Read the model definition and answer for the solid it produces. Units are mm, in the model's axes. A direction names the side the tool comes from. Round coordinates to 2 decimals unless told otherwise and drop trailing zeros. Write each loop counter-clockwise with the first axis right and the second up, starting at its lowest first coordinate (ties: lowest second). Pieces come first, ordered by that corner, then holes.
from build123d import *

# Parameters (mm, degrees)
BOSS_EXTRUDE1_DEPTH = 6
SKETCH2_W           = 6
SKETCH2_H           = 3


with BuildPart() as part:
    # Sketch1 → Boss-Extrude1 (new body)
    with BuildSketch(Plane(origin=(0, 0, 0), x_dir=(0, 0, -1), z_dir=(1, 0, 0))):
        Polygon((0, 5.773502692), (-5, 2.886751346), (-5, -2.886751346), (0, -5.773502692), (5, -2.886751346), (5, 2.886751346), align=None)
    extrude(amount=-BOSS_EXTRUDE1_DEPTH)

    # Sketch2 → Cut-Revolve4 (revolve, cut)
    with BuildSketch(Plane.XY):
        Polygon((0, 5), (-0.446581987, 5.773502692), (0, 5.773502692), align=None)
        with BuildLine():
            Line((-3.553418013, 5.773502692), (-4, 5))
            Line((-4, 5), (-5, 5))
            ThreePointArc((-5, 5), (-5.707106781, 4.707106781), (-6, 4))
            Line((-6, 4), (-6.773502692, 4))
            Line((-6.773502692, 4), (-6.773502692, 5.773502692))
            Line((-6.773502692, 5.773502692), (-3.553418013, 5.773502692))
        make_face()
        with Locations((-3, 1.5)):
            Rectangle(SKETCH2_W, SKETCH2_H)
    revolve(axis=Axis((-8.121993413, 0, 0), (1, 0, 0)), mode=Mode.SUBTRACT)


solid = part.part
Q1. Determine the mould class of faces 3 (the cylindrical face through (-3, -3, 0)), 4 (the conical face through (-3.894, 2.603, 4.483)), 5 (the flat face through (-1.972, -4.35, -2.465)), 6 (the flat face through (0, 0.1, -3.3)) for opening direction Y: pulls with the +Y half, pulls with the -Y half, needs draft (parallel to the pull), parting line crosses it, or undercut.
Verdict:
face 3: undercut
face 4: pulls with the +Y half
face 5: pulls with the -Y half
face 6: needs draft
Q2. Which of the six approach directions +Z, -Z, +X, -X, +Y, -Y give full straight-line access (tool end or side, diameter ignored) to faces 1 (the cylindrical face through (-4.51, -1.08, -4.88)), 2 (the flat face through (-1.972, -4.31, 2.535))?
Verdict:
face 1: -X
face 2: +Z, +X, -X, -Y
Q3. Straight lines are drawn through the part: probe 1 along Z at (x, y) = (-3.15, 0); probe 2 along Y at (x, z) = (-4.2, 2); probe 3 along Z at (x, y) = (-4.2, 2.25). For each, find the intervals that lie inside material, in ascending order.
Verdict:
probe 1: z = -5 to -3, 3 to 5
probe 2: y = -4.58 to -2.24, 2.24 to 4.58
probe 3: z = -4.47 to -1.98, 1.98 to 4.47
Q4. Section A-A (x = -2.4) is taken. Determine the outline of the cut face in (y, z), then the cut area to 3 significant figures.
Verdict:
outline: (-5.77, 0) - (-2.89, -5) - (2.89, -5) - (5.77, 0) - (2.89, 5) - (-2.89, 5) - close; hole circle Ø6 at (0, 0)
area: 58.3 mm2
